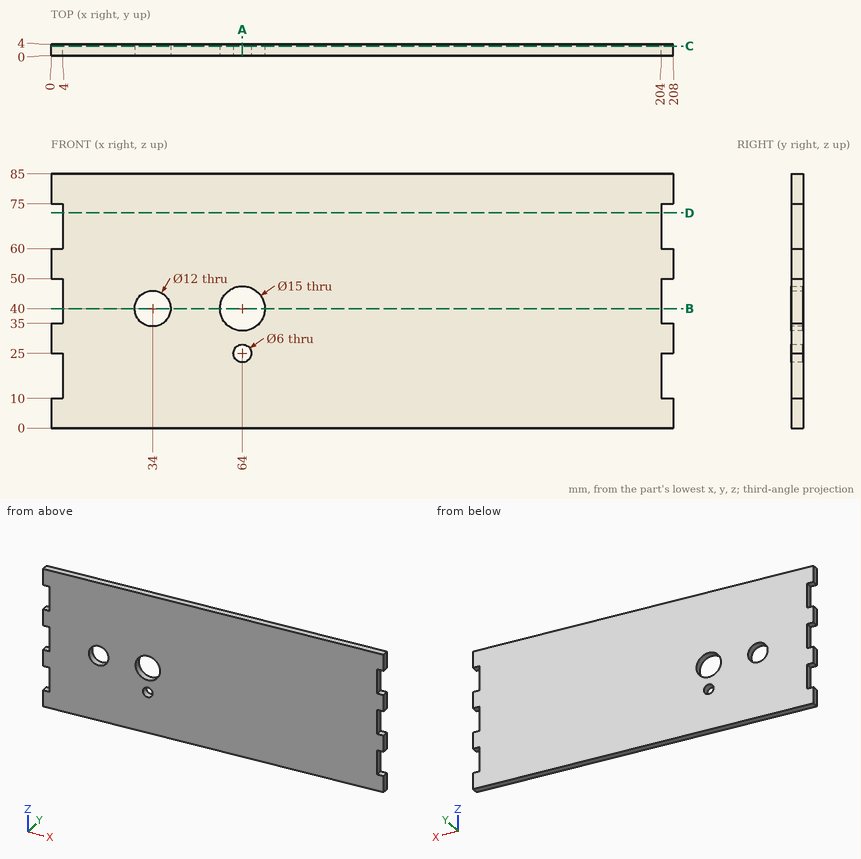
The figure shows three views and two pictorial views of one solid part (mm, origin at its lowest corner). Answer the questions. Round coordinates to 2 decimals unless told otherwise and drop trailing zeros. Write each loop counter-clockwise with the first axis right and the second up, starting at its lowest first coordinate (ties: lowest second). Pieces come first, ordered by that corner, then holes. Notation, with made-up numbers: (55, 21) -> (105, 21) arc R16 ccw to (105, 51) -> close; hole circle Ø5 at (59, -6.75). An arc over 180 degrees is marked (long way). Answer as a JSON object with one key per item and string values. Group by question number.
Q1. Straight lines are drawn through the part: line 1 along X through (y, z) = (0.95, 40); line 2 along Z through (x, y) = (62, 0.2); line 3 along X through (y, z) = (0.6, 25.5). For each, find the intervals that lie inside material, in ascending order.
Q2. Section A-A (x = 64) is taken. Write down the section's boundary in (y, z).
Q3. Section B-B (z = 40) is taken. Write down the section's boundary in (x, y), plus the area to 3 significant figures.
Q4. Section C-C (y = 3.3) is taken. Count the separate pieces of the cut face and the enclosed holes in it, plus the area to 3 significant figures.
Q5. Each of these flat-tipped pins is pushed along its axis until it touches: pin 1 Ø1.5 at (y, z) = (3, 70.5) entering from +X; pin 2 Ø2 at (y, z) = (3, 14) entering from -X. Where does it stop, or does it pass through?
Q6. Section D-D (z = 72) is taken. Write down the section's boundary in (x, y), plus the area to 3 significant figures.
Check values:
{
 "1": {"line 1": "4 to 28, 40 to 56.5, 71.5 to 204", "line 2": "0 to 22.76, 27.24 to 32.77, 47.23 to 85", "line 3": "0 to 61.04, 66.96 to 208"},
 "2": {"outline": "(0, 0) -> (4, 0) -> (4, 22) -> (0, 22) -> close; (0, 28) -> (4, 28) -> (4, 32.5) -> (0, 32.5) -> close; (0, 47.5) -> (4, 47.5) -> (4, 85) -> (0, 85) -> close"},
 "3": {"outline": "(4, 0) -> (28, 0) -> (28, 4) -> (4, 4) -> close; (40, 0) -> (56.5, 0) -> (56.5, 4) -> (40, 4) -> close; (71.5, 0) -> (204, 0) -> (204, 4) -> (71.5, 4) -> close", "area": "692 mm^2"},
 "4": {"separate pieces": "1", "enclosed holes": "3", "area": "17,000 mm^2"},
 "5": {"pin 1": "x = 204", "pin 2": "x = 4"},
 "6": {"outline": "(4, 0) -> (204, 0) -> (204, 4) -> (4, 4) -> close", "area": "800 mm^2"}
}
